```python
from build123d import *

# Parameters (mm, degrees)
F0_W          = 42
F0_H          = 42
F0_R          = 2.5
F0_R_2        = 15
F1_DEPTH      = 5
F2_DEPTH      = 5
F2_DEPTH_BACK = 30
F3_R          = 3
F4_DEPTH      = 50


with BuildPart() as f1:
    # F0 (on Top) → F1 (new body)
    with BuildSketch(Plane.XY):
        Rectangle(F0_W, F0_H)
        with Locations((-16.000001, -16.000001)):
            Circle(F0_R, mode=Mode.SUBTRACT)
        with Locations((16.000001, -16.000001)):
            Circle(F0_R, mode=Mode.SUBTRACT)
        Circle(F0_R_2, mode=Mode.SUBTRACT)
        with Locations((-16.000001, 16.000001)):
            Circle(F0_R, mode=Mode.SUBTRACT)
        with Locations((16.000001, 16.000001)):
            Circle(F0_R, mode=Mode.SUBTRACT)
    extrude(amount=F1_DEPTH)

    # F0 (on Top) → F2 (join, two sides)
    with BuildSketch(Plane.XY) as f2_sk:
        Polygon((49, 21), (21, 21), (21, -21), (49, -21), (49, -10), (31.125, -10), (31.125, 10), (49, 10), align=None)
    extrude(amount=F2_DEPTH)
    extrude(f2_sk.sketch, amount=-F2_DEPTH_BACK)

    # F3 (on face) → F4 (cut)
    with BuildSketch(Plane.XZ.offset(21)):
        with Locations((35.550814, -13.738759)):
            Circle(F3_R)
    extrude(amount=-F4_DEPTH, mode=Mode.SUBTRACT)


solid = f1.part
```
Build history of the part. All positions in model axes, mm. A direction names the side the tool comes from. Give positions to 0.01 mm unless a question says otherwise; leave off trailing zeros. Loops run counter-clockwise (first coordinate to the right, second up) from the corner with the lowest first, then second, coordinate; pieces in that order, holes last.
Item 1: Slice it at A-A, the plane x = 42. List the corners of the cut face in (y, z), and give its area (3 significant figures).
Answers follow:
outline: (-21, -30) - (-10, -30) - (-10, 5) - (-21, 5) - close; (10, -30) - (21, -30) - (21, 5) - (10, 5) - close
area: 770 mm2
Item 2: Pull direction Y, two halves, no side cores. Call faces 4 (the face through (29, -21, -8)), 5 (the face through (-14.85, -18.22, 2.46)), 6 (the face through (49, -16, -12)), 7 (the face through (-13.615, 16.751, 2.465)): released by +Y, released by -Y, zero draft, split by the parting line, or undercut.
Answers follow:
face 4: released by -Y
face 5: undercut
face 6: zero draft
face 7: undercut
Item 3: Slice it at B-B, the plane y = 0. List the corners of the cut face in (x, z) (3 decimals), and give its area (3 significant figures).
Answers follow:
outline: (-21, 0) - (-15, 0) - (-15, 5) - (-21, 5) - close; (15, 0) - (21, 0) - (21, -30) - (31.125, -30) - (31.125, 5) - (15, 5) - close
area: 414 mm2
Item 4: Flat gauge pins, fed straight in: pin 1 (12 mm diameter, centred on y = -5, z = -14.5, fed in from +X); pin 2 (21 mm diameter, centred on x = -9.5, y = -7, fed in from -Z); pin 3 (6 mm diameter, centred on y = 9.5, z = -10.5, fed in from -X); pin 4 (16 mm diameter, centred on y = 1.5, z = -10.5, fed in from +X) (3 decimals). Where does each tip first touch, or does it go through?
Answers follow:
pin 1: stops at x = 49
pin 2: stops at z = 0
pin 3: stops at x = 21
pin 4: stops at x = 31.125
Item 5: Slice it at D-D, the plane z = -12. List the corners of the cut face in (x, y) (3 decimals).
Answers follow:
outline: (21, -21) - (33.106, -21) - (33.106, -10) - (31.125, -10) - (31.125, 10) - (33.106, 10) - (33.106, 21) - (21, 21) - close; (37.996, -21) - (49, -21) - (49, -10) - (37.996, -10) - close; (37.996, 10) - (49, 10) - (49, 21) - (37.996, 21) - close
Item 6: Which spindle directions (+Z, -Z, +X, -X, +Y, -Y) get a long thin tool onto all of the face, cutting with end or side? Do faces 1 (the face through (40, 10, -12)), 2 (the face through (17.15, -18.22, 2.46)), 3 (the face through (21, 0, -15)). Say none if no direction does.
Answers follow:
face 1: +Z, -Z, +X
face 2: +Z, -Z
face 3: -Z, -X, +Y, -Y
Item 7: Slice it at C-C, the plane y = -11. List the corners of the cut face in (x, z).
Answers follow:
outline: (-21, 0) - (-10.2, 0) - (-10.2, 5) - (-21, 5) - close; (10.2, 0) - (21, 0) - (21, -30) - (49, -30) - (49, 5) - (10.2, 5) - close; hole circle Ø6 at (35.55, -13.74)
Item 8: Drill centre lines: line 1 (Y direction, x = 42, z = -23.5); line 2 (X direction, y = 14.5, z = -3); line 3 (X direction, y = 15.5, z = 3). Where is each one in solid material? Low to high.
Answers follow:
line 1: y = -21 to -10, 10 to 21
line 2: x = 21 to 49
line 3: x = -21 to -18.45, -13.55 to 13.55, 18.45 to 49
